```python
from build123d import *

# Parameters (mm, degrees)
BOSS_EXTRUDE1_DEPTH = 0.5
CIRPATTERN1_COUNT   = 7
SKETCH3_R           = 29.615
SKETCH3_R_2         = 28.415
BOSS_EXTRUDE2_DEPTH = 3.5
BOSS_EXTRUDE3_START = 3.5
SKETCH3_3_R         = 29.615
SKETCH3_3_R_2       = 28.415
SKETCH3_3_R_3       = 28.405
BOSS_EXTRUDE3_DEPTH = 0.4


with BuildPart() as part:
    # Sketch1 → Revolve1 (revolve)
    with BuildSketch(Plane.XY, mode=Mode.PRIVATE) as revolve1_sk:
        Polygon((-11.25, 8), (-12.25, 8), (-12.25, 1), (-23.75, 1), (-23.75, 5), (-28.405, 5), (-28.405, 3.5), (-25.25, 3.5), (-25.25, 0), (-10.25, 0), (-10.25, 1), (-11.25, 1), align=None)
    revolve(revolve1_sk.sketch.rotate(Axis((0, 0, 0), (0, 1, 0)), 270), axis=Axis((0, 0, 0), (0, 1, 0)))

    # Sketch2 → Boss-Extrude1 (add, symmetric)
    with BuildSketch(Plane.XY):
        Polygon((-12.25, 8), (-23.75, 5), (-24.25, 5), (-24.25, 1), (-23.75, 1), (-12.25, 1), (-11.75, 1), (-11.75, 8), align=None)
    boss_extrude1 = extrude(amount=BOSS_EXTRUDE1_DEPTH, both=True)

    # CirPattern1: Boss-Extrude1 ×7 about axis
    cirpattern1_axis = Axis((0, 0, 0), (0, 1, 0))
    for i in range(1, CIRPATTERN1_COUNT):
        add(boss_extrude1.rotate(cirpattern1_axis, i * 360 / CIRPATTERN1_COUNT))



with BuildPart() as body_2:
    # Sketch3 → Boss-Extrude2 (new body)
    with BuildSketch(Plane(origin=(0, 0, 0), x_dir=(1, 0, 0), z_dir=(0, 1, 0))):
        with Locations(Location((0, 0, 0), (0, 0, 270))):
            Circle(SKETCH3_R)
        with Locations(Location((0, 0, 0), (0, 0, 270))):
            Circle(SKETCH3_R_2, mode=Mode.SUBTRACT)
    extrude(amount=BOSS_EXTRUDE2_DEPTH)


with BuildPart() as part_1:
    add(part.part)

    add(body_2.part)  # Boss-Extrude3 merges body 2
    # Sketch3<3> → Boss-Extrude3 (add)
    # profile 1 of 2: a face of its own
    with BuildSketch(Plane(origin=(0, 0, 0), x_dir=(1, 0, 0), z_dir=(0, 1, 0)).offset(BOSS_EXTRUDE3_START)):
        with Locations(Location((0, 0, 0), (0, 0, 270))):
            Circle(SKETCH3_3_R)
        with Locations(Location((0, 0, 0), (0, 0, 270))):
            Circle(SKETCH3_3_R_2, mode=Mode.SUBTRACT)
    # profile 2 of 2: a face of its own
    with BuildSketch(Plane(origin=(0, 0, 0), x_dir=(1, 0, 0), z_dir=(0, 1, 0)).offset(BOSS_EXTRUDE3_START)):
        with Locations(Location((0, 0, 0), (0, 0, 270))):
            Circle(SKETCH3_3_R_2)
        with Locations(Location((0, 0, 0), (0, 0, 90))):
            Circle(SKETCH3_3_R_3, mode=Mode.SUBTRACT)
    extrude(amount=BOSS_EXTRUDE3_DEPTH)


solid = part_1.part
```
Model file for the job. Use its own axes, mm. A direction names the side the tool comes from. Round coordinates to 2 decimals unless told otherwise and drop trailing zeros. Use one line per item in the form item = value.
Item 1: Tool access for faces 1 (the face through (25.4, 3.5, -0.1)), 2 (the face through (-3, 1, -18)), 3 (the face through (10.006, 0.507, 2.222)): list every direction of +Z, -Z, +X, -X, +Y, -Y with a clear straight run to the whole face (end or side of a thin tool).
Returned:
face_1 = -Y
face_2 = +Y
face_3 = +Y, -Y
Item 2: Flat gauge pins, fed straight in: pin 1 Ø1 at (y, z) = (6, -19.5) entering from -X; pin 2 Ø6.5 at (x, z) = (16, 0) entering from +Y; pin 3 Ø1.5 at (y, z) = (1, 2.5) entering from -X. Where does each tip first touch, or does it go through?
Returned:
pin_1 = 3.82
pin_2 = 1
pin_3 = -29.56
Item 3: Drill centre lines: line 1 (X direction, y = 4.5, z = 0) (3 decimals); line 2 (X direction, y = 2.8, z = 0) (3 decimals); line 3 (X direction, y = 0.4, z = 0) (3 decimals). Where is each one in solid material? Low to high.
Returned:
line_1 = -28.405 to -11.25, 11.25 to 12.25, 23.75 to 28.405
line_2 = -29.615 to -28.415, -25.25 to -11.25, 11.25 to 12.25, 23.75 to 25.25, 28.415 to 29.615
line_3 = -29.615 to -28.415, -25.25 to -10.25, 10.25 to 25.25, 28.415 to 29.615
Item 4: Cut at B-B, the plane y = 1.75. Give the number of separate pieces and of enclosed holes in the cut face, and give its area (3 significant figures).
Returned:
separate_pieces = 2
enclosed_holes = 9
area = 604 mm^2
Item 5: Pull direction X, two halves, no side cores. Call faces 4 (the face through (26.5, 0, -11.1)), 5 (the face through (-11.66, 3.77, 13.82)), 6 (the face through (4.51, 3.77, 17.51)), 7 (the face through (16.15, 6.52, 7.77)): released by +X, released by -X, zero draft, split by the parting line, or undercut.
Returned:
face_4 = zero draft
face_5 = undercut
face_6 = undercut
face_7 = released by +X
